For this review, take the finished solid that the model builds, in its own axes (mm). Round coordinates to 2 decimals unless told otherwise and drop trailing zeros. Write each loop counter-clockwise with the first axis right and the second up, starting at its lowest first coordinate (ties: lowest second). Pieces come first, ordered by that corner, then holes. Notation, with made-up numbers: (27.25, 22.25) -> (79.25, 22.25) arc R20 ccw to (79.25, 34.25) -> close; hole circle Ø11 at (74, 34.25). An arc over 180 degrees is marked (long way). Answer in a Markdown table with one row per item.
Autodesk Inventor part; units mm, degrees
ref_plane "YZ Plane" through (0, 0, 0) normal (1, 0, 0) x (0, 1, 0)
ref_plane "XZ Plane" through (0, 0, 0) normal (0, 1, 0) x (-1, 0, 0)
ref_plane "XY Plane" through (0, 0, 0) normal (0, 0, 1) x (1, 0, 0)
sketch "Esquisse1" plane through (0, 0, 0) normal (0, 0, 1) x (1, 0, 0)
  line L0 (-50, -50) -> (50, -50)
  line L1 (50, -50) -> (50, 50)
  line L2 (50, 50) -> (-50, 50)
  line L3 (-50, 50) -> (-50, -50)
  line L4 (-50, -50) -> (50, 50) construction
  line L5 (50, -50) -> (-50, 50) construction
  line L6 (-38, 30) -> (-15, 30)
  line L7 (-15, 30) -> (-15, -14)
  line L8 (-15, -14) -> (-38, -14)
  line L9 (-38, -14) -> (-38, 30)
  line L10 (-38, 30) -> (-15, -14) construction
  line L11 (-15, 30) -> (-38, -14) construction
  line L12 (15, 30) -> (38, 30)
  line L13 (38, 30) -> (38, -14)
  line L14 (38, -14) -> (15, -14)
  line L15 (15, -14) -> (15, 30)
  line L16 (15, 30) -> (38, -14) construction
  line L17 (38, 30) -> (15, -14) construction
  circle A0 centre (-26.5, -36) radius 3
  circle A1 centre (26.5, -36) radius 3
  point P0 (0, 0)
  point P1 (-26.5, 8)
  point P2 (26.5, 8)
  point P3 (0, -50)
  dimension "d0" = 100
  dimension "d1" = 100
  dimension "d2" = 23
  dimension "d3" = 44
  dimension "d4" = 23
  dimension "d5" = 44
  dimension "d6" = 6
  dimension "d7" = 6
  dimension "d8" = 53
  dimension "d9" = 0
  dimension "d10" = 14
  dimension "d13" = 0
  dimension "d14" = 0
  dimension "d15" = 26.5
  dimension "d16" = 80
  dimension "d17" = 0
extrude "Extrusion1" add sketch "Esquisse1" along normal blind 5
properties part number "support_servo_Impression 3D"
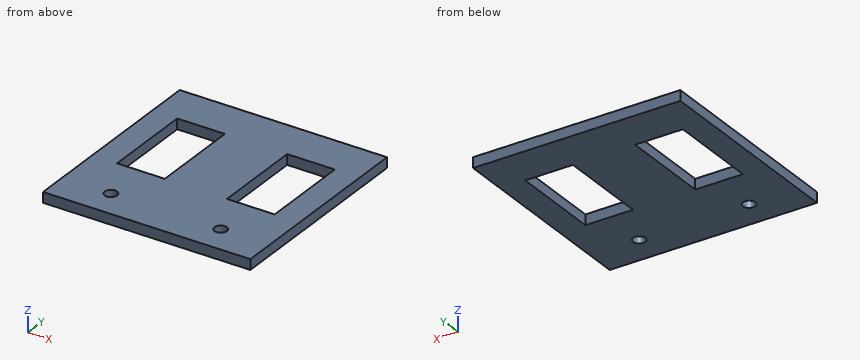
1) Clearance check with flat-ended pins moving along their axes: pin 1 Ø1 at (x, y) = (-0.5, -14.5) entering from -Z; pin 2 Ø3.5 at (x, y) = (26.5, -36) entering from -Z. State where each tip first meets the part, or that it passes through.
Solved:
| item | result |
|---|---|
| pin 1 | z = 0 |
| pin 2 | through |
2) Consider section A-A on x = 26.5. State the section outline as (y, z) points.
Solved:
| item | result |
|---|---|
| outline | (-50, 0) -> (-39, 0) -> (-39, 5) -> (-50, 5) -> close; (-33, 0) -> (-14, 0) -> (-14, 5) -> (-33, 5) -> close; (30, 0) -> (50, 0) -> (50, 5) -> (30, 5) -> close |
3) Consider section B-B on y = 26.5. State the section outline as (x, z) points.
Solved:
| item | result |
|---|---|
| outline | (-50, 0) -> (-38, 0) -> (-38, 5) -> (-50, 5) -> close; (-15, 0) -> (15, 0) -> (15, 5) -> (-15, 5) -> close; (38, 0) -> (50, 0) -> (50, 5) -> (38, 5) -> close |
4) Consider section C-C on z = 1.6. State the section outline as (x, y) points.
Solved:
| item | result |
|---|---|
| outline | (-50, -50) -> (50, -50) -> (50, 50) -> (-50, 50) -> close; hole (-38, -14) -> (-15, -14) -> (-15, 30) -> (-38, 30) -> close; hole circle Ø6 at (-26.5, -36); hole (15, -14) -> (38, -14) -> (38, 30) -> (15, 30) -> close; hole circle Ø6 at (26.5, -36) |
5) For line 1 (Y direction, x = -26.5, z = 1.4); line 2 (X direction, y = -3.5, z = 3.4); line 3 (Y direction, x = -29, z = 2.3), list the stretches that pass through material, from the lowest coordinate up. Write a range as [from, to].
Solved:
| item | result |
|---|---|
| line 1 | [-50, -39], [-33, -14], [30, 50] |
| line 2 | [-50, -38], [-15, 15], [38, 50] |
| line 3 | [-50, -37.66], [-34.34, -14], [30, 50] |
